from build123d import *

# Parameters (mm, degrees)
F0_W     = 126.9999751441
F0_H     = 127
F1_DEPTH = 127
F2_W     = 25.4
F2_H     = 28.2670979543
F3_DEPTH = 127
F5_DEPTH = 101.6


# Not quite as in the source:
# - a feature names something its author has since deleted; it is built from what else it names


with BuildPart() as f1:
    # F0 (on Front) → F1 (new body)
    with BuildSketch(Plane.XZ):
        with Locations((63.4999875721, -63.5)):
            Rectangle(F0_W, F0_H)
    extrude(amount=F1_DEPTH)

    # F2 (on face) → F3 (cut)
    with BuildSketch(Plane.XY):
        with Locations((114.2999751441, -112.8664510228)):
            Rectangle(F2_W, F2_H)
    extrude(amount=-F3_DEPTH, mode=Mode.SUBTRACT)

    # F4 (on face) → F5 (cut)
    with BuildSketch(Plane.XY):
        Polygon((25.3999751441, -25.4), (25.3999751441, -127), (101.5999751441, -127), (101.5999751441, -98.7329020457), (126.9999751441, -98.7329020457), (126.9999751441, -25.4), align=None)
    extrude(amount=-F5_DEPTH, mode=Mode.SUBTRACT)


solid = f1.part
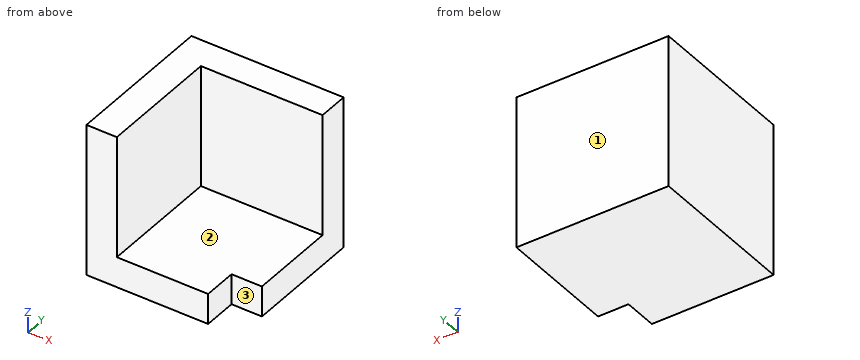
The model under review builds one solid part; all positions refer to its coordinate system, in mm. Face numbers are marked on the shaded views. A direction names the side the tool comes from. Give positions to 0.01 mm unless a question says otherwise; leave off trailing zeros. Write each loop counter-clockwise with the first axis right and the second up, starting at its lowest first coordinate (ties: lowest second). Pieces come first, ordered by that corner, then holes.
1. Wall thickness on L1, parallel to Y at x = 107.5, z = -73.5; L2, parallel to Z at x = 44.5, y = -62; L3, parallel to X at y = -35, z = -53.5: over which ranges is each line inside the solid? List them lowest first.
2. Tool access review of the marked faces 1, 2 and 3: name each direction out of +Z, -Z, +X, -X, +Y, -Y from which nothing blocks a thin tool from reaching the whole face with its end or side.
3. For P1, Ø12, axis at x = 98.5, z = -78, coming from the -Y side; P2, Ø20.5, axis at y = -110.5, z = -114, coming from the +X side; P3, Ø5, axis at y = -90, z = -58, coming from the +X side, all flat-tipped, find the tip position at first contact; note any pin that passes through.
4. Add section B-B, the plane z = -108. Write out the cut boundary in (x, y).
5. Add section A-A, the plane y = -62.5. Write out the cut boundary in (x, z).
Worked answers:
1. L1: y = -25.4 to 0
1. L2: z = -127 to -101.6
1. L3: x = 0 to 25.4
2. face 1: +Z, -Z, +X, -X, +Y
2. face 2: +Z, +X, -Y
2. face 3: +Z, -Z, +X, -Y
3. P1: stops at y = -25.4
3. P2: stops at x = 101.6
3. P3: stops at x = 25.4
4. outline: (0, -127) - (101.6, -127) - (101.6, -98.73) - (127, -98.73) - (127, 0) - (0, 0) - close
5. outline: (0, -127) - (127, -127) - (127, -101.6) - (25.4, -101.6) - (25.4, 0) - (0, 0) - close
